Autodesk Inventor part; units mm, degrees
ref_plane "YZ Plane" through (0, 0, 0) normal (1, 0, 0) x (0, 1, 0)
ref_plane "XZ Plane" through (0, 0, 0) normal (0, 1, 0) x (-1, 0, 0)
ref_plane "XY Plane" through (0, 0, 0) normal (0, 0, 1) x (1, 0, 0)
sketch "Sketch1" plane through (0, 0, 0) normal (0, 0, 1) x (1, 0, 0)
  line L0 (-9, -9) -> (9, -9) construction
  line L1 (9, -9) -> (9, 9) construction
  line L2 (9, 9) -> (-9, 9) construction
  line L3 (-9, 9) -> (-9, -9) construction
  line L4 (-9, -9) -> (9, 9) construction
  line L5 (9, -9) -> (-9, 9) construction
  circle A0 centre (-9, 9) radius 2
  circle A1 centre (9, 9) radius 2
  circle A2 centre (9, -9) radius 2
  circle A3 centre (-9, -9) radius 2
  line L6 (-13.4025, 9) -> (21.0308, 9) construction
  line L7 (-13.4025, -18) -> (21.0308, -18)
  line L8 (14, -14) -> (-14, -14)
  line L9 (-14, -14) -> (-14, 14)
  line L10 (-14, 14) -> (14, 14)
  line L11 (14, 14) -> (14, -14)
  line L12 (-14, 14) -> (14, 14)
  line L13 (14, 14) -> (14, -18)
  line L14 (14, -18) -> (-14, -18)
  line L15 (-14, -18) -> (-14, 14)
  point P0 (0, 0)
  dimension "d0" = 18
  dimension "d1" = 18
  dimension "d2" = 4
  dimension "d3" = 4
  dimension "d4" = 27
  dimension "d5" = 5
  dimension "d6" = 9
  dimension "d7" = 14
extrude "Extrusion1" add sketch "Sketch1" along normal blind 3
sketch "Sketch2" plane through (-14, -18, 0) normal (0, -1, 0) x (1, 0, 0)
  line L0 (0, 3) -> (28, 3)
  line L1 (28, 3) -> (28, 21)
  line L2 (28, 21) -> (0, 21)
  line L3 (0, 21) -> (0, 3)
  line L4 (0, 21) -> (28, 3) construction
  line L5 (5, 7.5) -> (23, 7.5) construction
  line L6 (23, 7.5) -> (23, 16.5) construction
  line L7 (23, 16.5) -> (5, 16.5) construction
  line L8 (5, 16.5) -> (5, 7.5) construction
  line L9 (5, 7.5) -> (23, 16.5) construction
  line L10 (23, 7.5) -> (5, 16.5) construction
  circle A0 centre (5, 16.5) radius 2
  circle A1 centre (23, 16.5) radius 2
  line L11 (5, 12) -> (23, 12) construction
  line L12 (14, 16.5) -> (14, 7.5) construction
  circle A2 centre (5, 7.5) radius 2
  circle A3 centre (23, 7.5) radius 2
  line L13 (0, 0) -> (28, 0)
  line L14 (28, 0) -> (28, 3)
  line L15 (0, 3) -> (28, 3)
  line L16 (0, 0) -> (0, 3)
  line L17 (0, 0) -> (28, 0)
  line L18 (28, 0) -> (28, 3)
  line L19 (28, 3) -> (0, 3)
  line L20 (0, 3) -> (0, 0)
  point P0 (14, 0)
  point P1 (14, 12)
  dimension "d11" = 18
  dimension "d12" = 18
  dimension "d13" = 9
  dimension "d14" = 4
  dimension "d15" = 4
extrude "Extrusion2" add sketch "Sketch2" against normal blind 3
sketch "Sketch4" plane through (-14, 14, 0) normal (-1, 0, 0) x (0, 0, 1)
  line L0 (3, -29) -> (3, 0)
  line L1 (21, -32) -> (21, -29)
  line L2 (0, 0) -> (0, -32)
  line L3 (3, -29) -> (21, -29)
  line L4 (21, -32) -> (21, -29)
  line L5 (3, 0) -> (3, -29)
  line L6 (0, 0) -> (3, 0)
  line L7 (0, -32) -> (21, -32)
  line L8 (3, 0) -> (21, -29)
  point P0 (0, -14)
  point P1 (3, -32)
  point P2 (3, 0)
  point P3 (21, -32)
  point P4 (3, 0)
extrude "Extrusion3" add sketch "Sketch4" along normal blind 3
mirror "Mirror1" about plane through (0, 0, 0) normal (1, 0, 0) of "Extrusion3"
sketch "Sketch5" plane through (-14, -18, 0) normal (0, -1, 0) x (1, 0, 0)
  circle A0 centre (5, 7.5) radius 2
  circle A1 centre (5, 7.5) radius 3
  point P0 (14, 0)
  dimension "d22" = 6
sketch "Sketch6" plane through (0, 0, 3) normal (0, 0, 1) x (1, 0, 0)
  circle A0 centre (-9, -9) radius 2
  circle A1 centre (-9, -9) radius 3
  point P0 (0, 0)
  dimension "d23" = 6
properties part number "Escuadra" material "ABS Plastic"
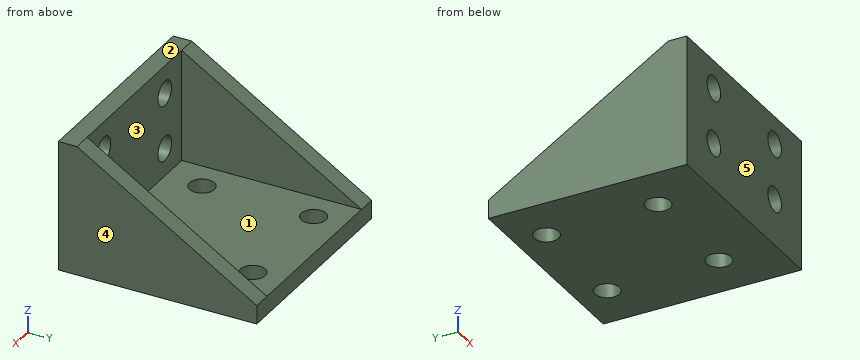
CAD build for the part. Positions are in the model's coordinates, mm. Face numbers are marked on the shaded views. A direction names the side the tool comes from. Coordinates: 2 decimals unless noted, no trailing zeros. Write each loop counter-clockwise with the first axis right and the second up, starting at its lowest first coordinate (ties: lowest second). Pieces come first, ordered by that corner, then holes.
(1) Drill centre lines: probe 1 along Z at (x, y) = (-9, -15.7); probe 2 along Y at (x, z) = (-9, 1.25); probe 3 along X at (y, z) = (-14, 6). Where is each one in solid material? Low to high.
(2) Cut at C-C, the plane y = -9. List the corners of the cut face in (x, z).
(3) 3-axis set-ups, long thin cutter, end or side, ignore diameter. For the marked faces 1 and 2: which of +Z, -Z, +X, -X, +Y, -Y reach the whole face in a straight line?
(4) Cut at B-B, the plane x = -9. List the corners of the cut face in (y, z), and give its area (3 significant figures).
(5) Cut at A-A, the plane z = 7.5. List the corners of the cut face in (x, y), and give its area (4 significant figures).
(6) Cut at D-D, the plane z = 2.5. List the corners of the cut face in (x, y).
(7) Two-plate mould, pull along X, no slides. Class the marked faces 3, 4 and 5: +X half, -X half, draft (parallel to the pull), parting line (faces both ways), or undercut.
(8) Flat gauge pins, fed straight in: pin 1 (1.5 mm diameter, centred on x = -8.5, y = 7.5, fed in from +Z); pin 2 (5.5 mm diameter, centred on x = -4, z = 14, fed in from +Y). Where does each tip first touch, or does it go through?
Geometry says:
1. probe 1: z = 0 to 5.5, 9.5 to 14.5, 18.5 to 21
1. probe 2: y = -18 to -11, -7 to 7, 11 to 14
1. probe 3: x = -17 to -14, 14 to 17
2. outline: (-17, 0) - (-11, 0) - (-11, 3) - (-14, 3) - (-14, 17.28) - (-17, 17.28) - close; (-7, 0) - (7, 0) - (7, 3) - (-7, 3) - close; (11, 0) - (17, 0) - (17, 17.28) - (14, 17.28) - (14, 3) - (11, 3) - close
3. face 1: +Z, +Y
3. face 2: +Z, +X, -X, +Y, -Y
4. outline: (-18, 0) - (-11, 0) - (-11, 3) - (-15, 3) - (-15, 5.5) - (-18, 5.5) - close; (-18, 9.5) - (-15, 9.5) - (-15, 14.5) - (-18, 14.5) - close; (-18, 18.5) - (-15, 18.5) - (-15, 21) - (-18, 21) - close; (-7, 0) - (7, 0) - (7, 3) - (-7, 3) - close; (11, 0) - (14, 0) - (14, 3) - (11, 3) - close
4. area: 102 mm2
5. outline: (-17, -18) - (-11, -18) - (-11, -15) - (-14, -15) - (-14, 6.75) - (-17, 6.75) - close; (-7, -18) - (7, -18) - (7, -15) - (-7, -15) - close; (11, -18) - (17, -18) - (17, 6.75) - (14, 6.75) - (14, -15) - (11, -15) - close
5. area: 208.5 mm2
6. outline: (-17, -18) - (17, -18) - (17, 14) - (-17, 14) - close; hole circle Ø4 at (-9, -9); hole circle Ø4 at (-9, 9); hole circle Ø4 at (9, -9); hole circle Ø4 at (9, 9)
7. face 3: undercut
7. face 4: +X half
7. face 5: draft
8. pin 1: stops at z = 3
8. pin 2: stops at y = -15
